from build123d import *

# Parameters (mm, degrees)
SKETCH128_R  = 1.5
PAD102_DEPTH = 50
SKETCH126_R  = 1.7
PAD100_DEPTH = 50
SKETCH124_R  = 1.7
PAD098_DEPTH = 50
SKETCH127_R  = 1.5
PAD101_DEPTH = 20
PAD078_DEPTH = 4
SKETCH109_R  = 1.5
PAD082_DEPTH = 5
SKETCH106_R  = 1.5
PAD077_DEPTH = 5


with BuildPart() as topscrewcutouts:
    # Sketch128 → Pad102 (new body)
    with BuildSketch(Plane.XY):
        with Locations((0, 79)):
            Circle(SKETCH128_R)
        with Locations((-10, 47.5)):
            Circle(SKETCH128_R)
        with Locations((10, 47.5)):
            Circle(SKETCH128_R)
        with Locations((-10, 24.5)):
            Circle(SKETCH128_R)
        with Locations((10, 24.5)):
            Circle(SKETCH128_R)
        with Locations((0, 59)):
            Circle(SKETCH128_R)
    extrude(amount=PAD102_DEPTH)


with BuildPart() as screwcutout:
    # Sketch126 → Pad100 (new body)
    with BuildSketch(Plane(origin=(0, 70, 0), x_dir=(1, 0, 0), z_dir=(0, 0, 1))):
        with Locations((0, -2.75)):
            Circle(SKETCH126_R)
    extrude(amount=PAD100_DEPTH)


with BuildPart() as pad098:
    # Sketch124 → Pad098 (new body)
    with BuildSketch(Plane(origin=(0, 40, 0), x_dir=(1, 0, 0), z_dir=(0, 0, 1))):
        with Locations((0, -2.75)):
            Circle(SKETCH124_R)
    extrude(amount=PAD098_DEPTH)


with BuildPart() as cutouts:
    # Sketch127 → Pad101 (new body)
    with BuildSketch(Plane.XZ.offset(-74)):
        with Locations((0, 22)):
            Circle(SKETCH127_R)
    extrude(amount=-PAD101_DEPTH)

    # Fusion004020004: union ScrewCutout, Pad098
    add(screwcutout.part)
    add(pad098.part)


with BuildPart() as obj1:
    # Sketch102 → Pad078 (new body, symmetric)
    with BuildSketch(Plane.YZ):
        Polygon((17, 19), (27, 19), (27, 24.35), (30.5, 24.35), (30.5, 19), (34, 19), (34, 24.35), (40.5, 24.35), (40.5, 19), (50, 19), (50, 24.35), (53.5, 24.35), (53.5, 19), (64, 19), (64, 24.35), (70.5, 24.35), (70.5, 19), (86, 19), (86, 26), (92, 26), (90, 28), (24.551897, 28), align=None)
    extrude(amount=PAD078_DEPTH, both=True)


with BuildPart() as centermount:
    # Sketch109 → Pad082 (new body)
    with BuildSketch(Plane.XZ.offset(-50)):
        with BuildLine():
            Line((-12.04196, 20.5), (12.04196, 20.5))
            ThreePointArc((12.04196, 20.5), (15.250889, 18.010509), (18, 21.000021))
            Line((18, 25.171573), (18, 21.000021))
            Line((15.171573, 28), (18, 25.171573))
            Line((-15.171573, 28), (15.171573, 28))
            Line((-18, 25.171573), (-15.171573, 28))
            Line((-18, 21), (-18, 25.171573))
            ThreePointArc((-18, 21), (-15.250879, 18.010508), (-12.04196, 20.5))
        make_face()
        with Locations((15, 21)):
            Circle(SKETCH109_R, mode=Mode.SUBTRACT)
        with Locations((-15, 21)):
            Circle(SKETCH109_R, mode=Mode.SUBTRACT)
    extrude(amount=PAD082_DEPTH)


with BuildPart() as cut007019010:
    # Sketch106 → Pad077 (new body)
    with BuildSketch(Plane.XZ.offset(-27)):
        with BuildLine():
            Line((-12.04196, 20.5), (12.04196, 20.5))
            ThreePointArc((12.04196, 20.5), (15.250889, 18.010509), (18, 21.000021))
            Line((18, 25.171573), (18, 21.000021))
            Line((15.171573, 28), (18, 25.171573))
            Line((-15.171573, 28), (15.171573, 28))
            Line((-18, 25.171573), (-15.171573, 28))
            Line((-18, 21), (-18, 25.171573))
            ThreePointArc((-18, 21), (-15.250879, 18.010508), (-12.04196, 20.5))
        make_face()
        with Locations((15, 21)):
            Circle(SKETCH106_R, mode=Mode.SUBTRACT)
        with Locations((-15, 21)):
            Circle(SKETCH106_R, mode=Mode.SUBTRACT)
    extrude(amount=PAD077_DEPTH)

    # Fusion004020002: union obj1, CenterMount
    add(obj1.part)
    add(centermount.part)

    # Cut007019009: cut Cutouts
    add(cutouts.part, mode=Mode.SUBTRACT)

    # Cut007019010: cut TopScrewCutouts
    add(topscrewcutouts.part, mode=Mode.SUBTRACT)


solid = cut007019010.part
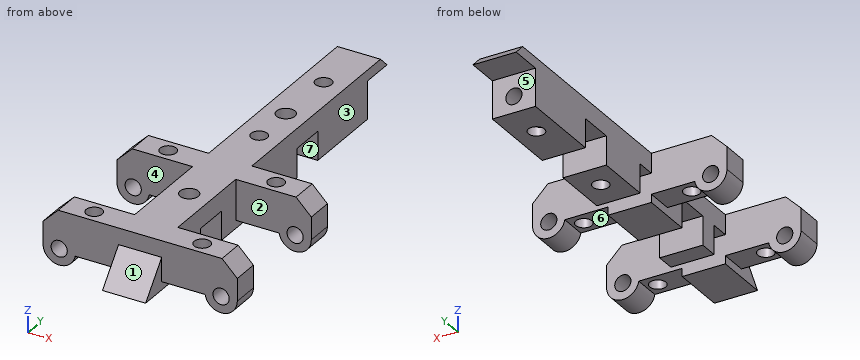
Source: CAD feature listing. Evaluate the final solid. Frame: model axes, mm. Face numbers are marked on the shaded views. A direction names the side the tool comes from. Coordinates: 2 decimals unless noted, no trailing zeros. Loops run counter-clockwise (first coordinate to the right, second up) from the corner with the lowest first, then second, coordinate; pieces in that order, holes last. Notation, with made-up numbers: (20.5, 45.25) - (70.5, 45.25) arc R11 ccw to (70.5, 58.25) - close; hole circle Ø8 at (-24, 60). An arc over 180 degrees is marked (long way). Return JSON: item names as keys, results as strings.
Q1. Mould query, pull axis Y, two halves, no side actions, for the marked faces 1, 2 and 3. Classes: released by +Y, released by -Y, zero draft, split by the parting line, or undercut.
Results:
{"face 1": "released by -Y", "face 2": "undercut", "face 3": "zero draft"}
Q2. Section B-B, the plane y = 67.25. Return loops of the section in (x, z), plus the area to 3 significant figures.
Results:
{"outline": "(-4, 24.35) - (-1.7, 24.35) - (-1.7, 28) - (-4, 28) - close; (1.7, 24.35) - (4, 24.35) - (4, 28) - (1.7, 28) - close", "area": "16.8 mm2"}
Q3. Contact query for flat-ended pins moving along their axis: P1, Ø5, axis at x = 10, y = 24.5, coming from the -Z side; P2, Ø4, axis at x = 8.5, y = 25, coming from the -Z side; P3, Ø12, axis at x = -3, y = 34, coming from the -Z side. Output: stop coordinate, or through.
Results:
{"P1": "z = 19.34", "P2": "z = 20.5", "P3": "z = 19"}
Q4. Section D-D, the plane y = 75. Return loops of the section in (x, z), plus the area to 3 significant figures.
Results:
{"outline": "(-4, 19) - (4, 19) - (4, 28) - (-4, 28) - close; hole circle Ø3 at (0, 22)", "area": "64.9 mm2"}
Q5. Section A-A, the plane x = -10. Return loops of the section in (y, z).
Results:
{"outline": "(22, 20.5) - (23, 20.5) - (23, 28) - (22, 28) - close; (26, 20.5) - (27, 20.5) - (27, 28) - (26, 28) - close; (45, 20.5) - (46, 20.5) - (46, 28) - (45, 28) - close; (49, 20.5) - (50, 20.5) - (50, 28) - (49, 28) - close"}
Q6. Section C-C, the plane y = 24.5. Return loops of the section in (x, z).
Results:
{"outline": "(-18, 21) arc R3 ccw to (-12.04, 20.5) - (-11.5, 20.5) - (-11.5, 28) - (-15.17, 28) - (-18, 25.17) - close; (-8.5, 20.5) - (-4, 20.5) - (-4, 19) - (4, 19) - (4, 20.5) - (8.5, 20.5) - (8.5, 28) - (-8.5, 28) - close; (11.5, 20.5) - (12.04, 20.5) arc R3 ccw to (18, 21) - (18, 25.17) - (15.17, 28) - (11.5, 28) - close; hole circle Ø3 at (-15, 21); hole circle Ø3 at (15, 21)"}
Q7. Access query for the marked faces 4, 5, 6 and 7. Directions: +Z, -Z, +X, -X, +Y, -Y. A direction counts if a zero-diameter tool reaches every point of the face in a straight line with its end or side. Return the directions, or none.
Results:
{"face 4": "+Z, -Z, -X", "face 5": "-Z, +X, -X, +Y", "face 6": "-Z, +Y, -Y", "face 7": "-Z, +X, -X"}
Q8. Material intervals for line 1 along X through (y, z) = (24.5, 23.75); line 2 along X through (y, z) = (79, 26.8); line 3 along Y through (x, z) = (5.5, 24), sorted ascending.
Results:
{"line 1": "-18 to -11.5, -8.5 to 8.5, 11.5 to 18", "line 2": "-4 to -1.5, 1.5 to 4", "line 3": "22 to 27, 45 to 50"}
